Geometry: see drawing. Coordinates: mm, zero at the bounding-box minimum. A direction names the side the tool comes from. Coordinates: 2 decimals unless noted, no trailing zeros. Order: outer loops, then holes, each group sorted by start corner. A loop starts at its lowest first (then second) coordinate and runs counter-clockwise, first axis right, second up. Notation, with made-up numbers: (20, 16.25) -> (31, 16.25) arc R33 cw to (31, 51.25) -> close; hole circle Ø4 at (6, 9). An arc over 180 degrees is marked (long way). Use one line per item in the form item = value.
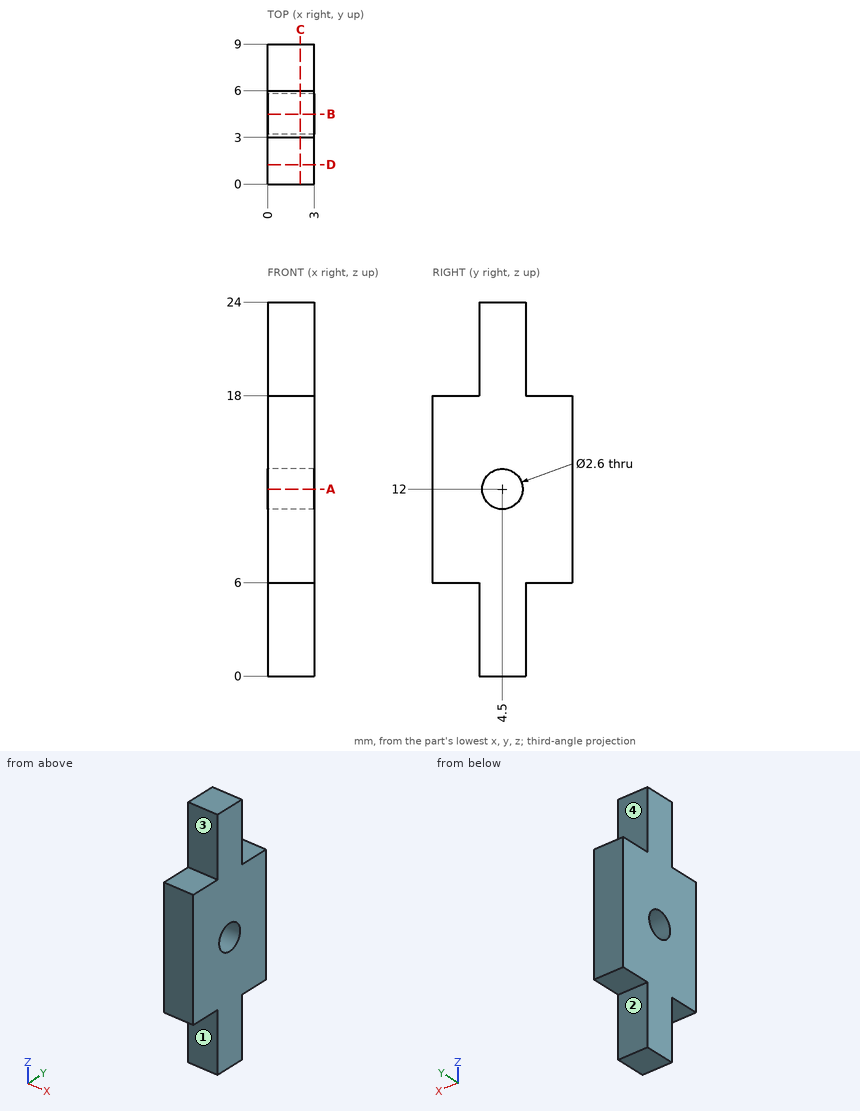
1) Section A-A, the plane z = 12. Output: boundary loops of the cut face in (x, y).
Results found:
outline = (0, 0) -> (3, 0) -> (3, 3.2) -> (0, 3.2) -> close; (0, 5.8) -> (3, 5.8) -> (3, 9) -> (0, 9) -> close
2) Material intervals for probe 1 along Y at (x, z) = (2.2, 12); probe 2 along Z at (x, y) = (0.9, 5); probe 3 along Y at (x, z) = (0.4, 22.75), sorted ascending. Write a range as from..to.
Results found:
probe_1 = 0..3.2, 5.8..9
probe_2 = 0..10.8, 13.2..24
probe_3 = 3..6
3) Section C-C, the plane x = 2.1. Output: boundary loops of the cut face in (y, z).
Results found:
outline = (0, 6) -> (3, 6) -> (3, 0) -> (6, 0) -> (6, 6) -> (9, 6) -> (9, 18) -> (6, 18) -> (6, 24) -> (3, 24) -> (3, 18) -> (0, 18) -> close; hole circle Ø2.6 at (4.5, 12)
4) Access query for the marked faces 1, 2, 3 and 4. Directions: +Z, -Z, +X, -X, +Y, -Y. A direction counts if a zero-diameter tool reaches every point of the face in a straight line with its end or side. Return the directions, or none.
Results found:
face_1 = -Z, +X, -X, -Y
face_2 = -Z, +X, -X, +Y
face_3 = +Z, +X, -X, -Y
face_4 = +Z, +X, -X, +Y
5) Contact query for flat-ended pins moving along their axis: P1, Ø1.5, axis at x = 1, y = 1, coming from the +Z side; P2, Ø0.9, axis at x = 1, y = 7.5, coming from the -Z side; P3, Ø1.5, axis at x = 1.5, z = 3, coming from the +Y side. Output: stop coordinate, or through.
Results found:
P1 = 18
P2 = 6
P3 = 6
6) Section D-D, the plane y = 1.25. Output: boundary loops of the cut face in (x, z), and give its area (3 significant figures).
Results found:
outline = (0, 6) -> (3, 6) -> (3, 18) -> (0, 18) -> close
area = 36.0 mm2
7) Section B-B, the plane y = 4.5. Output: boundary loops of the cut face in (x, z).
Results found:
outline = (0, 0) -> (3, 0) -> (3, 10.7) -> (0, 10.7) -> close; (0, 13.3) -> (3, 13.3) -> (3, 24) -> (0, 24) -> close
